from build123d import *

# Parameters (mm, degrees)
SKICA1_R                 = 5.25
P_IDAT_VYSUNUT_M1_DEPTH  = 5
ZAOBLIT1_R               = 4
P_IDAT_VYSUNUT_M3_DEPTH  = 5
SKICA5_R                 = 4.25
SKICA5_R_2               = 1.75
P_IDAT_VYSUNUT_M4_DEPTH  = 1
SKICA8_R                 = 1.05
ODEBRAT_VYSUNUT_M3_DEPTH = 6
ODEBRAT_VYSUNUT_M4_DEPTH = 7
SKICA2_R                 = 1.75
ODEBRAT_VYSUNUT_M5_DEPTH = 10
SKICA10_R                = 3.5
ODEBRAT_VYSUNUT_M6_DEPTH = 3
ODEBRAT_START            = 50
SKICA11_R                = 0.75
ODEBRAT_VYSUNUT_M7_DEPTH = 10
P_IDAT_VYSUNUT_M5_DEPTH  = 10
P_IDAT_VYSUNUT_M6_DEPTH  = 8
ZAOBLIT2_R               = 2
ODEBRAT_VYSUNUT_M8_DEPTH = 7


with BuildPart() as part:
    # Skica1 → Přidat vysunutím1 (new body, symmetric)
    with BuildSketch(Plane.XY):
        with BuildLine():
            Line((0, 0), (0, 16))
            Line((0, 16), (24, 16))
            Line((24, 16), (24, 0))
            Line((24, 0), (29, 0))
            Line((29, 0), (97.312746067, 39.440382331))
            ThreePointArc((97.312746067, 39.440382331), (105.473420704, 36.802978572), (112.433277726, 41.81425579))
            Line((112.433277726, 41.81425579), (195.687578405, 27.134276321))
            ThreePointArc((195.687578405, 27.134276321), (209.374429572, 27.607666525), (196.674905514, 32.733686604))
            Line((196.674905514, 32.733686604), (113.420604835, 47.413666074))
            ThreePointArc((113.420604835, 47.413666074), (102.174688824, 55.511016714), (94.812746067, 43.77050935))
            Line((94.812746067, 43.77050935), (29, 5.773502692))
            Line((29, 5.773502692), (29, 21))
            Line((29, 21), (-5, 21))
            Line((-5, 21), (-5, 0))
            Line((-5, 0), (0, 0))
        make_face()
        with Locations((104, 46.188021535)):
            Circle(SKICA1_R, mode=Mode.SUBTRACT)
    extrude(amount=P_IDAT_VYSUNUT_M1_DEPTH, both=True)

    # Zaoblit1
    zaoblit1_edges = [part.edges().sort_by_distance(p)[0] for p in [
        (-5, 21, 0),
    ]]
    fillet(zaoblit1_edges, radius=ZAOBLIT1_R)

    # Skica4 → Přidat vysunutím3 (add, symmetric)
    with BuildSketch(Plane.XY):
        Polygon((29, 21), (66.969109888, 27.694978507), (59.37284323, 23.309271907), (29, 17.953720164), align=None)
    extrude(amount=P_IDAT_VYSUNUT_M3_DEPTH, both=True)

    # Skica5 → Přidat vysunutím4 (add)
    with BuildSketch(Plane.XY.offset(5)):
        with Locations((202.480775301, 28.823203768)):
            Circle(SKICA5_R)
        with Locations((202.480775301, 28.823203768)):
            Circle(SKICA5_R_2, mode=Mode.SUBTRACT)
    extrude(amount=P_IDAT_VYSUNUT_M4_DEPTH)

    # Skica8 → Odebrat vysunutím3 (cut)
    with BuildSketch(Plane.XZ):
        with Locations((-1.5, 0)):
            Circle(SKICA8_R)
        with Locations((25.5, 0)):
            Circle(SKICA8_R)
    extrude(amount=-ODEBRAT_VYSUNUT_M3_DEPTH, mode=Mode.SUBTRACT)

    # Skica9 → Odebrat vysunutím4 (cut)
    with BuildSketch(Plane.XY.offset(5)):
        Polygon((24, 16), (29, 16), (29, 13), (24, 8), align=None)
    extrude(amount=-ODEBRAT_VYSUNUT_M4_DEPTH, mode=Mode.SUBTRACT)

    # Skica2 → Odebrat vysunutím5 (cut)
    with BuildSketch(Plane.XY.offset(5)):
        with Locations((202.480775301, 28.823203768)):
            Circle(SKICA2_R)
    extrude(amount=-ODEBRAT_VYSUNUT_M5_DEPTH, mode=Mode.SUBTRACT)

    # Skica10 → Odebrat vysunutím6 (cut)
    with BuildSketch(Plane(origin=(0, 0, -5), x_dir=(-1, 0, 0), z_dir=(0, 0, -1))):
        with Locations((-202.480775301, 28.823203768)):
            Circle(SKICA10_R)
    extrude(amount=-ODEBRAT_VYSUNUT_M6_DEPTH, mode=Mode.SUBTRACT)

    # Skica11 → Odebrat vysunutím7 (cut)
    with BuildSketch(Plane(origin=(0, 0, 0), x_dir=(1, 0, 0), z_dir=(0, 1, 0)).offset(ODEBRAT_START)):
        with Locations((103.960302418, 0)):
            Circle(SKICA11_R)
    extrude(amount=ODEBRAT_VYSUNUT_M7_DEPTH, mode=Mode.SUBTRACT)

    # Skica12 → Přidat vysunutím5 (add)
    with BuildSketch(Plane.XY.offset(5)):
        with BuildLine():
            Line((195.687578405, 27.134276321), (195.687578405, 16.823203768))
            Line((195.687578405, 16.823203768), (209.480775301, 16.823203768))
            Line((209.480775301, 16.823203768), (209.480775301, 28.823203768))
            ThreePointArc((209.480775301, 28.823203768), (203.331546047, 21.875096894), (195.687578405, 27.134276321))
        make_face()
    extrude(amount=-P_IDAT_VYSUNUT_M5_DEPTH)

    # Skica13 → Přidat vysunutím6 (add)
    with BuildSketch(Plane.XY.offset(5)):
        Polygon((201.084176853, 20.823203768), (204.084176853, 20.823203768), (206.834176853, 16.823203768), (198.334176853, 16.823203768), align=None)
    extrude(amount=P_IDAT_VYSUNUT_M6_DEPTH)

    # Zaoblit2
    zaoblit2_edges = [part.edges().sort_by_distance(p)[0] for p in [
        (209.480775301, 16.823203768, 0),
        (195.687578405, 16.823203768, 0),
    ]]
    fillet(zaoblit2_edges, radius=ZAOBLIT2_R)

    # Skica14 → Odebrat vysunutím8 (cut)
    with BuildSketch(Plane.XY.offset(5)):
        Polygon((59.37284323, 23.309271907), (66.969109888, 27.694978507), (61.786216453, 26.781094556), (54.189949795, 22.395387956), align=None)
    extrude(amount=-ODEBRAT_VYSUNUT_M8_DEPTH, mode=Mode.SUBTRACT)


solid = part.part
Check sheet for the modelled part. Datum: model origin and axes. Units: mm. A direction names the side the tool comes from. Round coordinates to 2 decimals unless told otherwise and drop trailing zeros. Order: outer loops, then holes, each group sorted by start corner. A loop starts at its lowest first (then second) coordinate and runs counter-clockwise, first axis right, second up.
Q1. Draft check along Y on faces 5 (the face through (27, 11, 2)), 6 (the face through (203, 16.823, 4)), 7 (the face through (-5, 9, 0)), 8 (the face through (58.04, 24.62, 1.55)). Enter one of: pulls with the +Y half, pulls with the -Y half, needs draft (parallel to the pull), parting line crosses it, or undercut.
Filled sheet:
face 5: undercut
face 6: pulls with the -Y half
face 7: needs draft
face 8: undercut
Q2. Depth check by flat-ended pin: P1, Ø1.7, axis at x = 25.5, z = 0, coming from the -Y side; P2, Ø1.5, axis at x = 26, y = 11, coming from the +Z side; P3, Ø3, axis at x = 202.5, z = 3.5, coming from the -Y side; P4, Ø3, axis at x = 202.48, y = 28.82, coming from the -Z side. Enter the tip coordinate at first touch or a pass-through.
Filled sheet:
P1: stops at y = 6
P2: stops at z = 5
P3: stops at y = 16.82
P4: passes through
Q3. Cross-section at A-A, the plane x = 42. Enter the section's corners in (y, z), plus the area to 3 significant figures.
Filled sheet:
outline: (7.51, -5) - (13.28, -5) - (13.28, 5) - (7.51, 5) - close; (20.25, -5) - (23.29, -5) - (23.29, 5) - (20.25, 5) - close
area: 88.2 mm2
Q4. Scan lines: L1, parallel to X at y = 12.5, z = -4; L2, parallel to Y at x = 20, z = -1.25; L3, parallel to Y at x = 107, z = -1.5. Record each from-to range of solid material in increasing order.
Filled sheet:
L1: x = -5 to 0, 24 to 29, 40.65 to 50.65
L2: y = 16 to 21
L3: y = 37.17 to 41.88, 50.5 to 55.2
Q5. Cross-section at B-B, the plane z = 10. Enter the section's corners in (x, y).
Filled sheet:
outline: (198.33, 16.82) - (206.83, 16.82) - (204.08, 20.82) - (201.08, 20.82) - close
Q6. Cross-section at C-C, the plane x = 154. Enter the section's corners in (y, z).
Filled sheet:
outline: (34.48, -5) - (40.26, -5) - (40.26, 5) - (34.48, 5) - close
Q7. Set-up check for faces 1 (the face through (0, 8, 0)), 2 (the face through (155.63, 39.97, 0.07)), 3 (the face through (15.9, 16.4, 5)), 4 (the face through (203.4, 27, 6)): record each of +Z, -Z, +X, -X, +Y, -Y from which the full face is reachable in a straight line by a thin tool's end or side.
Filled sheet:
face 1: +Z, -Z, -Y
face 2: +Z, -Z, +Y
face 3: +Z, -X, +Y, -Y
face 4: +Z, +X, -X, +Y
